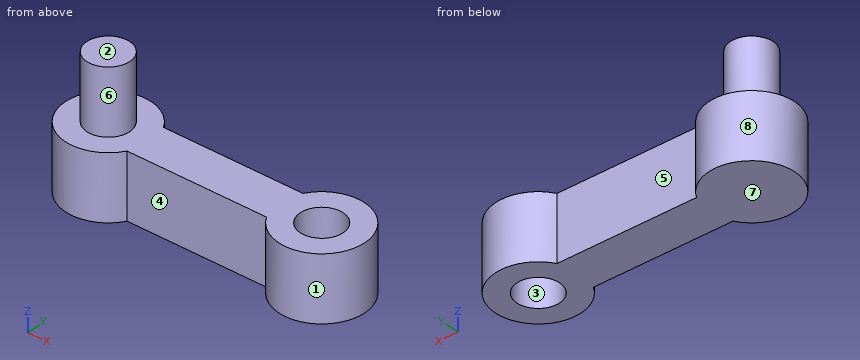
```python
from build123d import *

# Parameters (mm, degrees)
BOSS_EXTRUDE1_DEPTH = 3
SKETCH3_R           = 1
BOSS_EXTRUDE2_DEPTH = 3
SKETCH4_R           = 1
CUT_EXTRUDE1_DEPTH  = 3


with BuildPart() as part:
    # Sketch2 → Boss-Extrude1 (new body)
    with BuildSketch(Plane.XY):
        with BuildLine():
            Line((-36.5050045, 13.800340042), (-29.969106115, 13.800340042))
            ThreePointArc((-29.969106115, 13.800340042), (-26.237055307, 12.800340042), (-29.969106115, 11.800340042))
            Line((-29.969106115, 11.800340042), (-36.5050045, 11.800340042))
            ThreePointArc((-36.5050045, 11.800340042), (-40.237055307, 12.800340042), (-36.5050045, 13.800340042))
        make_face()
    extrude(amount=BOSS_EXTRUDE1_DEPTH)

    # Sketch3 → Boss-Extrude2 (add)
    with BuildSketch(Plane.XY.offset(3)):
        with Locations((-38.237055307, 12.800340042)):
            Circle(SKETCH3_R)
    extrude(amount=BOSS_EXTRUDE2_DEPTH)

    # Sketch4 → Cut-Extrude1 (cut)
    with BuildSketch(Plane(origin=(0, 0, 0), x_dir=(-1, 0, 0), z_dir=(0, 0, -1))):
        with Locations((28.237055307, 12.800340042)):
            Circle(SKETCH4_R)
    extrude(amount=-CUT_EXTRUDE1_DEPTH, mode=Mode.SUBTRACT)


solid = part.part
```
Verification items for the finished model (mm, model axes). Face numbers are marked on the shaded views. A direction names the side the tool comes from. Give positions to 0.01 mm unless a question says otherwise; leave off trailing zeros. Order: outer loops, then holes, each group sorted by start corner. A loop starts at its lowest first (then second) coordinate and runs counter-clockwise, first axis right, second up. Notation, with made-up numbers: M 14,-23 L 73,-23 A24 ccw 73,4 Z; hole C 19,69.25 d7. An arc over 180 degrees is marked long. Answer in a Markdown table with one row per item. Add a question column.
Item 1: Section check B-B, the plane y = 12.55. Enter the section's corners in (x, z), and give its area (3 significant figures).
Item 2: Tool access check on the marked faces 4, 5, 6, 7 and 8. Record the directions out of +Z, -Z, +X, -X, +Y, -Y that give a thin tool (end or side, any length) a straight path to the whole face; none if there is none.
Item 3: Section check A-A, the plane x = -29. Enter the section's corners in (y, z).
Item 4: Scan lines: probe 1 along Z at (x, y) = (-26.75, 13.6); probe 2 along X at (y, z) = (11, 0.8); probe 3 along Y at (x, z) = (-33.25, 2.7). Record each from-to range of solid material in increasing order. Write a range as from..to.
Item 5: Gauge pin test, flat ends, axial feed: pin 1 (1.5 mm diameter, centred on x = -33, z = 2, fed in from -Y); pin 2 (1 mm diameter, centred on x = -37, z = 2, fed in from -Y); pin 3 (0.9 mm diameter, centred on x = -31.5, z = 2, fed in from +Y). Record the tip position at first contact, or that the pin passes through.
Item 6: Section check D-D, the plane x = -36. Enter the section's corners in (y, z).
Item 7: Mould release check, pull along Y, two halves, no side actions. Record for the marked faces 1, 2 and 3: released by +Y, released by -Y, zero draft, split by the parting line, or undercut.
Item 8: Section check C-C, the plane z = 1.85. Enter the section's corners in (x, y) (3 decimals), and give its area (3 significant figures).
Filled sheet:
| question | item | result |
|---|---|---|
| 1 | outline | M -40.22,0 L -29.21,0 L -29.21,3 L -37.27,3 L -37.27,6 L -39.21,6 L -39.21,3 L -40.22,3 Z; M -27.27,0 L -26.25,0 L -26.25,3 L -27.27,3 Z |
| 1 | area | 41.9 mm^2 |
| 2 | face 4 | +Z, -Z, -Y |
| 2 | face 5 | +Z, -Z, +Y |
| 2 | face 6 | +Z |
| 2 | face 7 | -Z, +X, -X, +Y, -Y |
| 2 | face 8 | +Z, -Z |
| 3 | outline | M 10.95,0 L 12.15,0 L 12.15,3 L 10.95,3 Z; M 13.45,0 L 14.65,0 L 14.65,3 L 13.45,3 Z |
| 4 | probe 1 | z = 0..3 |
| 4 | probe 2 | x = -39.11..-37.37, -29.11..-27.37 |
| 4 | probe 3 | y = 11.8..13.8 |
| 5 | pin 1 | stops at y = 11.8 |
| 5 | pin 2 | stops at y = 10.94 |
| 5 | pin 3 | stops at y = 13.8 |
| 6 | outline | M 11.8,0 L 13.8,0 L 13.8,3 L 11.8,3 Z |
| 7 | face 1 | split by the parting line |
| 7 | face 2 | zero draft |
| 7 | face 3 | undercut |
| 8 | outline | M -36.505,11.8 L -29.969,11.8 A2 ccw long -29.969,13.8 L -36.505,13.8 A2 ccw long Z; hole C -28.237,12.8 d2 |
| 8 | area | 34.3 mm^2 |
